Verification items for the finished model (mm, model axes). A direction names the side the tool comes from. Give positions to 0.01 mm unless a question says otherwise; leave off trailing zeros. Order: outer loops, then holes, each group sorted by start corner. A loop starts at its lowest first (then second) coordinate and runs counter-clockwise, first axis right, second up.
from build123d import *

# Parameters (mm, degrees)
F0_W     = 50.8
F0_H     = 76.2
F1_DEPTH = 19.05
F3_R     = 6.35
F4_DEPTH = 19.05
F2_W     = 11.43
F2_H     = 17.78
F5_DEPTH = 8.89


with BuildPart() as f1:
    # F0 (on Top) → F1 (new body, symmetric)
    with BuildSketch(Plane.XY):
        Rectangle(F0_W, F0_H)
    extrude(amount=F1_DEPTH, both=True)

    # F3 (on face) → F4 (cut)
    with BuildSketch(Plane.XY.offset(19.05)):
        Polygon((-17.78, 38.1), (-17.78, 30.48), (-25.4, 30.48), (-25.4, -12.7), (-13.97, -12.7), (-13.97, -30.48), (13.97, -30.48), (13.97, -12.7), (25.4, -12.7), (25.4, 30.48), (17.78, 30.48), (17.78, 38.1), align=None)
        with Locations((0, -19.05)):
            Circle(F3_R, mode=Mode.SUBTRACT)
    extrude(amount=-F4_DEPTH, mode=Mode.SUBTRACT)

    # F2 (on face) → F5 (cut)
    with BuildSketch(Plane.XY.offset(19.05)):
        with Locations((19.685, -21.59)):
            Rectangle(F2_W, F2_H)
        with Locations((-19.685, -21.59)):
            Rectangle(F2_W, F2_H)
    extrude(amount=-F5_DEPTH, mode=Mode.SUBTRACT)


solid = f1.part
(1) Section check A-A, the plane z = 4.5. Enter the section's corners in (x, y), then the cut area to 3 significant figures.
Solved:
outline: (-25.4, -38.1) - (25.4, -38.1) - (25.4, -12.7) - (13.97, -12.7) - (13.97, -30.48) - (-13.97, -30.48) - (-13.97, -12.7) - (-25.4, -12.7) - close; (-25.4, 30.48) - (-17.78, 30.48) - (-17.78, 38.1) - (-25.4, 38.1) - close; circle Ø12.7 at (0, -19.05); (17.78, 30.48) - (25.4, 30.48) - (25.4, 38.1) - (17.78, 38.1) - close
area: 1,040 mm2
(2) Go/stop test with flat-tipped pins: pin 1 (9.5 mm diameter, centred on x = 4.5, z = 10.5, fed in from +Y); pin 2 (4 mm diameter, centred on x = -4, y = 5.5, fed in from +Z); pin 3 (8 mm diameter, centred on x = -13, y = -21.5, fed in from +Z). Record where each tip stops, or that it passes through.
Solved:
pin 1: stops at y = -12.7
pin 2: stops at z = 0
pin 3: stops at z = 10.16
(3) Set-up check for faces 4 (the flat face through (-13.97, -21, 5)), 5 (the flat face through (22, 30.48, 10)), 6 (the flat face through (-20, -21, 10.16)), 7 (the flat face through (20, -21, 10.16)): record each of +Z, -Z, +X, -X, +Y, -Y from which the full face is reachable in a straight line by a thin tool's end or side.
Solved:
face 4: +Z, +Y
face 5: +Z, +X, -X
face 6: +Z, -X
face 7: +Z, +X
(4) Scan lines: line 1 (X direction, y = -19.5, z = 9); line 2 (X direction, y = 32, z = 4.5); line 3 (Y direction, x = 21.5, z = 16.5). Record each from-to range of solid material in increasing order.
Solved:
line 1: x = -25.4 to -13.97, -6.33 to 6.33, 13.97 to 25.4
line 2: x = -25.4 to -17.78, 17.78 to 25.4
line 3: y = -38.1 to -30.48, 30.48 to 38.1
(5) Release check for a two-part mould opening along X. For faces 1 (the flat face through (0, -38.1, 0)), 2 (the flat face through (25.4, -1, -4)), 3 (the flat face through (13.97, -22, 5)) record: pulls with the +X half, pulls with the -X half, needs draft (parallel to the pull), parting line crosses it, or undercut.
Solved:
face 1: needs draft
face 2: pulls with the +X half
face 3: undercut
(6) Section check C-C, the plane y = -19.05. Enter the section's corners in (x, z).
Solved:
outline: (-25.4, -19.05) - (25.4, -19.05) - (25.4, 10.16) - (13.97, 10.16) - (13.97, 0) - (6.35, 0) - (6.35, 19.05) - (-6.35, 19.05) - (-6.35, 0) - (-13.97, 0) - (-13.97, 10.16) - (-25.4, 10.16) - close
(7) Section check B-B, the plane x = -19. Enter the section's corners in (y, z), then the cut area to 3 significant figures.
Solved:
outline: (-38.1, -19.05) - (38.1, -19.05) - (38.1, 19.05) - (30.48, 19.05) - (30.48, 0) - (-12.7, 0) - (-12.7, 10.16) - (-30.48, 10.16) - (-30.48, 19.05) - (-38.1, 19.05) - close
area: 1,920 mm2
(8) Section check D-D, the plane z = 14. Enter the section's corners in (x, y), then the cut area to 3 significant figures.
Solved:
outline: (-25.4, -38.1) - (25.4, -38.1) - (25.4, -30.48) - (-25.4, -30.48) - close; (-25.4, 30.48) - (-17.78, 30.48) - (-17.78, 38.1) - (-25.4, 38.1) - close; circle Ø12.7 at (0, -19.05); (17.78, 30.48) - (25.4, 30.48) - (25.4, 38.1) - (17.78, 38.1) - close
area: 630 mm2
